Part model, mm, in its own coordinate system. Face numbers are marked on the shaded views. A direction names the side the tool comes from. Give positions to 0.01 mm unless a question says otherwise; leave off trailing zeros. Order: outer loops, then holes, each group sorted by start corner. A loop starts at its lowest first (then second) coordinate and runs counter-clockwise, first axis right, second up.
Autodesk Inventor part; units mm, degrees
ref_plane "YZ Plane" through (0, 0, 0) normal (1, 0, 0) x (0, 1, 0)
ref_plane "XZ Plane" through (0, 0, 0) normal (0, 1, 0) x (-1, 0, 0)
ref_plane "XY Plane" through (0, 0, 0) normal (0, 0, 1) x (1, 0, 0)
sketch "スケッチ1" plane through (0, 0, 0) normal (1, 0, 0) x (0, 1, 0)
  line L0 (8.9, -3) -> (8.9, -9)
  line L1 (8.9, -9) -> (7, -9)
  line L2 (7, -9) -> (7, -44)
  line L3 (7, -44) -> (0, -44)
  line L4 (0, -44) -> (0, 0)
  line L5 (8.9, -3) -> (7.7, -3)
  line L6 (7.7, -3) -> (7.7, 0)
  line L7 (7.7, 0) -> (0, 0)
  dimension "d0" = 8.9
  dimension "d1" = 3
  dimension "d2" = 9
  dimension "d4" = 7.7
  dimension "d5" = 7
  dimension "d10" = 35
revolve "回転1" add sketch "スケッチ1" angle 360 about axis through (0, 0, -44) along (0, 0, 1)
chamfer "面取り1" distance 0.2 angle 45 1 edges at (0, -7.7, 0)
properties part number "AP6MS54G" material "ABS プラスチック"
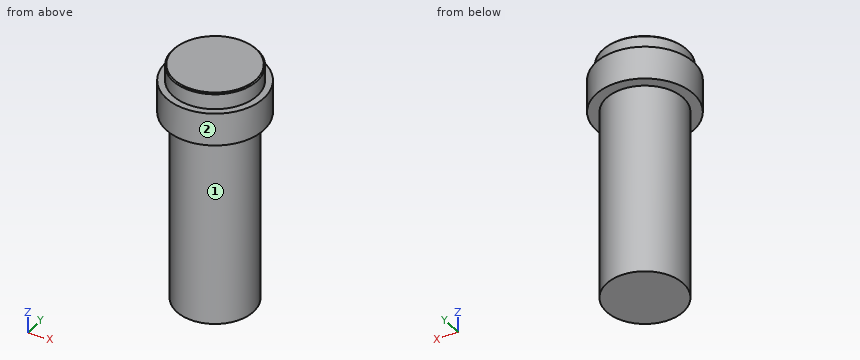
Item 1: Drill centre lines: probe 1 along Y at (x, z) = (5.5, -6); probe 2 along Z at (x, y) = (6.75, -3); probe 3 along Z at (x, y) = (-2.25, 8.25). Where is each one in solid material? Low to high.
Item 2: Band-saw the part on B-B on z = -28. List the corners of the cut face in (x, y).
Item 3: Drop flat-ended pins along their axis: P1, Ø8, axis at y = -4.5, z = -14, coming from the -X side; P2, Ø5, axis at x = -3.5, z = -39, coming from the +Y side; P3, Ø1, axis at x = -3, z = -18, coming from the -Y side. Give the stop position or say it passes through.
Item 4: Which spindle directions (+Z, -Z, +X, -X, +Y, -Y) get a long thin tool onto all of the face, cutting with end or side? Do the marked faces 1 and 2. Say none if no direction does.
Item 5: Band-saw the part on A-A on y = 0. List the corners of the cut face in (x, z), plus the area to 3 significant figures.
Working result:
1. probe 1: y = -7 to 7
1. probe 2: z = -9 to 0
1. probe 3: z = -9 to -3
2. outline: circle Ø14 at (0, 0)
3. P1: stops at x = -6.98
3. P2: stops at y = 6.93
3. P3: stops at y = -6.54
4. face 1: -Z
4. face 2: +Z, -Z
5. outline: (-8.9, -9) - (-7, -9) - (-7, -44) - (7, -44) - (7, -9) - (8.9, -9) - (8.9, -3) - (7.7, -3) - (7.7, -0.2) - (7.5, 0) - (-7.5, 0) - (-7.7, -0.2) - (-7.7, -3) - (-8.9, -3) - close
5. area: 643 mm2
